Model file for the job. Use its own axes, mm. A direction names the side the tool comes from. Give positions to 0.01 mm unless a question says otherwise; leave off trailing zeros. Order: outer loops, then holes, each group sorted by start corner. A loop starts at its lowest first (then second) coordinate and runs counter-clockwise, first axis right, second up. Notation, with made-up numbers: (-25.75, 18.25) -> (20.25, 18.25) arc R24 cw to (20.25, 57.25) -> close; hole circle Ø11 at (23, -27.75). An arc over 180 degrees is marked (long way). Use CSV: the item, a comma, the result in double quotes. Start each with the question number.
1. Cut at C-C on z = -15. List the corners of the cut face in (x, y).
2. 3-axis set-ups, long thin cutter, end or side, ignore diameter. For faces 1 (the cylindrical face through (-48.217, 1.972, 90.936)), 2 (the flat face through (47.718, 6, 53)), 3 (the cylindrical face through (-56.12, 1.97, 54.6)), 4 (the flat face through (-63.956, 2, -47)), 5 (the flat face through (61.77, 1.97, 57.78)): which of +Z, -Z, +X, -X, +Y, -Y reach the whole face in a straight line?
3. Drop flat-ended pins along their axis: pin 1 (2.5 mm diameter, centred on y = 6.5, z = 70.5, fed in from +X); pin 2 (4 mm diameter, centred on y = 7.5, z = 41, fed in from -X); pin 3 (2.5 mm diameter, centred on x = -59.25, z = -56.34, fed in from -Y); pin 4 (4 mm diameter, centred on x = -13, y = 7, fed in from -Z). Give the stop position or say it passes through.
4. Cut at B-B on z = 19. List the corners of the cut face in (x, y), then the cut area to 3 significant figures.
5. Cut at A-A on y = 6.5. List the corners of the cut face in (x, z), then the cut area to 3 significant figures.
6. Wall check: line 1 (X direction, y = 8.75, z = 82); line 2 (Z direction, x = 28.5, y = 6); line 3 (Z direction, x = 18.5, y = 2). Give the ranges that are in metal, low to high. Write a range as from..to.
```python
from build123d import *

# Parameters (mm, degrees)
SKETCH1_R           = 1.7
BOSS_EXTRUDE2_DEPTH = 4
SKETCH4_W           = 95.436014614
SKETCH4_H           = 75.892817578
SKETCH4_W_2         = 91.839367952
SKETCH4_H_2         = 73.032685056
BOSS_EXTRUDE5_DEPTH = 5


with BuildPart() as part:
    # Sketch1 → Boss-Extrude2 (new body)
    with BuildSketch(Plane(origin=(0, 0, 0), x_dir=(1, 0, 0), z_dir=(0, 1, 0))):
        with BuildLine():
            Line((55, -97.276480298), (-55, -97.276480298))
            Line((-55, -97.276480298), (-55, -95.836582418))
            ThreePointArc((-55, -95.836582418), (-56.256563164, -92.16237407), (-59.499935661, -90.027124011))
            Line((-59.499935661, -90.027124011), (-64.123335896, -88.833312587))
            ThreePointArc((-64.123335896, -88.833312587), (-67.366708393, -86.698062528), (-68.623271557, -83.02385418))
            Line((-68.623271557, -83.02385418), (-68.623271557, -64.477065442))
            ThreePointArc((-68.623271557, -64.477065442), (-67.538437873, -61.035969674), (-64.676224862, -58.839212772))
            Line((-64.676224862, -58.839212772), (-58.952120675, -56.75485206))
            ThreePointArc((-58.952120675, -56.75485206), (-56.08783115, -54.555127217), (-55.005078353, -51.109754923))
            Line((-55.005078353, -51.109754923), (-55.050338054, -13.624867313))
            ThreePointArc((-55.050338054, -13.624867313), (-53.526628764, -9.622267963), (-49.722190465, -7.65535648))
            Line((-49.722190465, -7.65535648), (-19.667476765, -4.268691216))
            ThreePointArc((-19.667476765, -4.268691216), (-16.201629955, -2.651477365), (-14.417006114, 0.731212762))
            Line((-14.417006114, 0.731212762), (-10.931405786, 22.181381875))
            ThreePointArc((-10.931405786, 22.181381875), (-12.283485184, 27.031277264), (-16.853724474, 29.143744262))
            Line((-16.853724474, 29.143744262), (-63.956383701, 29.143744262))
            Line((-63.956383701, 29.143744262), (-63.956383701, 64.872936213))
            Line((-63.956383701, 64.872936213), (-53.943716214, 64.872936213))
            Line((-53.943716214, 64.872936213), (-53.943716214, 38.878522988))
            Line((-53.943716214, 38.878522988), (53.943716214, 38.878522988))
            Line((53.943716214, 38.878522988), (53.943716214, 64.872936213))
            Line((53.943716214, 64.872936213), (63.956383701, 64.872936213))
            Line((63.956383701, 64.872936213), (63.956383701, 29.143744262))
            Line((63.956383701, 29.143744262), (16.853724474, 29.143744262))
            ThreePointArc((16.853724474, 29.143744262), (12.283485184, 27.031277264), (10.931405786, 22.181381875))
            Line((10.931405786, 22.181381875), (14.417006114, 0.731212762))
            ThreePointArc((14.417006114, 0.731212762), (16.201629955, -2.651477365), (19.667476765, -4.268691216))
            Line((19.667476765, -4.268691216), (49.722190465, -7.65535648))
            ThreePointArc((49.722190465, -7.65535648), (53.526628764, -9.622267963), (55.050338054, -13.624867313))
            Line((55.050338054, -13.624867313), (55.005078353, -51.109754923))
            ThreePointArc((55.005078353, -51.109754923), (56.08783115, -54.555127217), (58.952120675, -56.75485206))
            Line((58.952120675, -56.75485206), (64.676224862, -58.839212772))
            ThreePointArc((64.676224862, -58.839212772), (67.538437873, -61.035969674), (68.623271557, -64.477065442))
            Line((68.623271557, -64.477065442), (68.623271557, -83.02385418))
            ThreePointArc((68.623271557, -83.02385418), (67.366708393, -86.698062528), (64.123335896, -88.833312587))
            Line((64.123335896, -88.833312587), (59.499935661, -90.027124011))
            ThreePointArc((59.499935661, -90.027124011), (56.256563164, -92.16237407), (55, -95.836582418))
            Line((55, -95.836582418), (55, -97.276480298))
        make_face()
        with Locations(Location((-59.25, 56.33553485, 0), (0, 0, 270))):
            Circle(SKETCH1_R, mode=Mode.SUBTRACT)
        with Locations(Location((-59.25, 34.83553485, 0), (0, 0, 270))):
            Circle(SKETCH1_R, mode=Mode.SUBTRACT)
        with Locations(Location((59.25, 34.83553485, 0), (0, 0, 270))):
            Circle(SKETCH1_R, mode=Mode.SUBTRACT)
        with Locations(Location((59.25, 56.33553485, 0), (0, 0, 270))):
            Circle(SKETCH1_R, mode=Mode.SUBTRACT)
        with Locations(Location((0, 19.658684952, 0), (0, 0, 270))):
            Circle(SKETCH1_R, mode=Mode.SUBTRACT)
        with Locations(Location((61.535021632, -64.239476302, 0), (0, 0, 270))):
            Circle(SKETCH1_R, mode=Mode.SUBTRACT)
        with Locations(Location((-8.660254038, 4.658684952, 0), (0, 0, 270))):
            Circle(SKETCH1_R, mode=Mode.SUBTRACT)
        with Locations(Location((8.660254038, 4.658684952, 0), (0, 0, 270))):
            Circle(SKETCH1_R, mode=Mode.SUBTRACT)
        with Locations(Location((61.535021632, -81.039476302, 0), (0, 0, 270))):
            Circle(SKETCH1_R, mode=Mode.SUBTRACT)
        with Locations(Location((-61.535021632, -81.039476302, 0), (0, 0, 270))):
            Circle(SKETCH1_R, mode=Mode.SUBTRACT)
        with Locations(Location((-61.535021632, -64.239476302, 0), (0, 0, 270))):
            Circle(SKETCH1_R, mode=Mode.SUBTRACT)
        with Locations(Location((-49.365711, -13.675658, 0), (0, 0, 270))):
            Circle(SKETCH1_R, mode=Mode.SUBTRACT)
        with Locations(Location((-49.365711, -92.189056, 0), (0, 0, 270))):
            Circle(SKETCH1_R, mode=Mode.SUBTRACT)
        with Locations(Location((49.365711, -92.189056, 0), (0, 0, 270))):
            Circle(SKETCH1_R, mode=Mode.SUBTRACT)
        with Locations(Location((49.365711, -13.675658, 0), (0, 0, 270))):
            Circle(SKETCH1_R, mode=Mode.SUBTRACT)
    extrude(amount=BOSS_EXTRUDE2_DEPTH)

    # Sketch4 → Boss-Extrude5 (add)
    with BuildSketch(Plane(origin=(0, 4, 0), x_dir=(1, 0, 0), z_dir=(0, 1, 0))):
        with Locations((0, -52.932357)):
            Rectangle(SKETCH4_W, SKETCH4_H)
        with Locations((0, -52.932357)):
            Rectangle(SKETCH4_W_2, SKETCH4_H_2, mode=Mode.SUBTRACT)
    extrude(amount=BOSS_EXTRUDE5_DEPTH)


solid = part.part
```
Verdict:
1,outline,"(-12.1, 0) -> (12.1, 0) -> (12.1, 4) -> (-12.1, 4) -> close"
2,face 1,"+Y, -Y"
2,face 2,"+Z, -Z, +X, +Y"
2,face 3,"-X, +Y, -Y"
2,face 4,"-Z, -X, +Y, -Y"
2,face 5,"+X, +Y, -Y"
3,pin 1,"x = 47.72"
3,pin 2,"x = -47.72"
3,pin 3,"through"
3,pin 4,"z = 14.99"
4,outline,"(-55.04, 0) -> (55.04, 0) -> (55.04, 4) -> (47.72, 4) -> (47.72, 9) -> (45.92, 9) -> (45.92, 4) -> (-45.92, 4) -> (-45.92, 9) -> (-47.72, 9) -> (-47.72, 4) -> (-55.04, 4) -> close"
4,area,"458 mm^2"
5,outline,"(-47.72, 14.99) -> (47.72, 14.99) -> (47.72, 90.88) -> (-47.72, 90.88) -> close; hole (-45.92, 16.42) -> (45.92, 16.42) -> (45.92, 89.45) -> (-45.92, 89.45) -> close"
5,area,"536 mm^2"
6,line 1,"-47.72..-45.92, 45.92..47.72"
6,line 2,"14.99..16.42, 89.45..90.88"
6,line 3,"-38.88..-29.14, 4.02..97.28"
